Check sheet for the modelled part. Datum: model origin and axes. Units: mm. Face numbers are marked on the shaded views. A direction names the side the tool comes from. Round coordinates to 2 decimals unless told otherwise and drop trailing zeros. Write each loop counter-clockwise with the first axis right and the second up, starting at its lowest first coordinate (ties: lowest second). Pieces come first, ordered by that corner, then holes.
Item 1: Set-up check for the marked faces 1, 2, 3 and 4: record each of +Z, -Z, +X, -X, +Y, -Y from which the full face is reachable in a straight line by a thin tool's end or side.
Item 2: Section check B-B, the plane z = 10. State how many separate pieces and enclosed holes the cut face has, plus the area to 3 significant figures.
Item 3: Section check C-C, the plane y = -13. Record the cut outline in (x, z), plus the area to 3 significant figures.
Item 4: Material ranges on line 1 along Z through (x, y) = (24, 8.3); line 2 along Y through (x, z) = (-11, 18.75); line 3 along Y through (x, z) = (-6.5, 9.5), recorded low to high.
Item 5: Section check D-D, the plane x = 16. Record the cut outline in (y, z), plus the area to 3 significant figures.
Item 6: Release check for a two-part mould opening along Y. For the marked faces 5, 6 and 7 record: pulls with the +Y half, pulls with the -Y half, needs draft (parallel to the pull), parting line crosses it, or undercut.
Item 7: Section check A-A, the plane x = 24. Record the cut outline in (y, z), plus the area to 3 significant figures.
Item 8: Depth check by flat-ended pin: pin 1 (5.5 mm diameter, centred on x = 24, z = 9.5, fed in from -Y); pin 2 (10 mm diameter, centred on y = 11.5, z = 14, fed in from -X); pin 3 (2 mm diameter, centred on y = 18, z = 7.5, fed in from -X); pin 4 (5.5 mm diameter, centred on x = 24.5, z = 8.5, fed in from +Y). Enter the tip coordinate at first touch or a pass-through.
from build123d import *

# Parameters (mm, degrees)
SKETCH1_W           = 6.8
SKETCH1_H           = 2
SKETCH1_W_2         = 40
SKETCH1_H_2         = 39
BOSS_EXTRUDE1_DEPTH = 20
SKETCH2_R           = 4.5
BOSS_EXTRUDE2_DEPTH = 2
SKETCH3_R           = 5
BOSS_EXTRUDE3_DEPTH = 1.9
SKETCH4_R           = 3
BOSS_EXTRUDE4_DEPTH = 4
SKETCH5_R           = 10
BOSS_EXTRUDE5_DEPTH = 2
SKETCH6_R           = 2
CUT_EXTRUDE1_DEPTH  = 10
SKETCH7_R           = 2
CUT_EXTRUDE2_DEPTH  = 10
CUT_EXTRUDE3_DEPTH  = 5


with BuildPart() as part:
    # Sketch1 → Boss-Extrude1 (new body)
    with BuildSketch(Plane.XY):
        with Locations((-23.4, 7.722986842)):
            Rectangle(SKETCH1_W, SKETCH1_H)
        with Locations((0, -1.777013158)):
            Rectangle(SKETCH1_W_2, SKETCH1_H_2)
        with Locations((23.4, 7.722986842)):
            Rectangle(SKETCH1_W, SKETCH1_H)
    extrude(amount=BOSS_EXTRUDE1_DEPTH)

    # Sketch2 → Boss-Extrude2 (add)
    with BuildSketch(Plane(origin=(0, 17.722986842, 0), x_dir=(1, 0, 0), z_dir=(0, 1, 0))):
        with Locations(Location((-10, -10, 0), (0, 0, 180))):
            Circle(SKETCH2_R)
    extrude(amount=BOSS_EXTRUDE2_DEPTH)

    # Sketch3 → Boss-Extrude3 (add)
    with BuildSketch(Plane(origin=(0, 17.722986842, 0), x_dir=(1, 0, 0), z_dir=(0, 1, 0))):
        with Locations((-10, -10)):
            Circle(SKETCH3_R)
    extrude(amount=BOSS_EXTRUDE3_DEPTH)

    # Sketch4 → Boss-Extrude4 (add)
    with BuildSketch(Plane(origin=(0, 19.722986842, 0), x_dir=(1, 0, 0), z_dir=(0, 1, 0))):
        with Locations(Location((-10, -10, 0), (0, 0, 180))):
            Circle(SKETCH4_R)
    extrude(amount=BOSS_EXTRUDE4_DEPTH)

    # Sketch5 → Boss-Extrude5 (add)
    with BuildSketch(Plane(origin=(0, 23.722986842, 0), x_dir=(1, 0, 0), z_dir=(0, 1, 0))):
        with Locations(Location((-10, -10, 0), (0, 0, 180))):
            Circle(SKETCH5_R)
    extrude(amount=BOSS_EXTRUDE5_DEPTH)

    # Sketch6 → Cut-Extrude1 (cut)
    with BuildSketch(Plane(origin=(0, 8.722986842, 0), x_dir=(1, 0, 0), z_dir=(0, 1, 0))):
        with Locations(Location((24, -4, 0), (0, 0, 180))):
            Circle(SKETCH6_R)
        with Locations(Location((24, -16, 0), (0, 0, 180))):
            Circle(SKETCH6_R)
    extrude(amount=-CUT_EXTRUDE1_DEPTH, mode=Mode.SUBTRACT)

    # Sketch7 → Cut-Extrude2 (cut)
    with BuildSketch(Plane(origin=(0, 8.722986842, 0), x_dir=(1, 0, 0), z_dir=(0, 1, 0))):
        with Locations(Location((-24, -4, 0), (0, 0, 180))):
            Circle(SKETCH7_R)
        with Locations(Location((-24, -16, 0), (0, 0, 180))):
            Circle(SKETCH7_R)
    extrude(amount=-CUT_EXTRUDE2_DEPTH, mode=Mode.SUBTRACT)

    # Sketch8 → Cut-Extrude3 (cut)
    with BuildSketch(Plane(origin=(0, 25.722986842, 0), x_dir=(1, 0, 0), z_dir=(0, 1, 0))):
        with BuildLine():
            ThreePointArc((-18, -10), (-17, -11), (-16, -10))
            Line((-16, -10), (-18, -10))
        make_face()
        with BuildLine():
            Line((-18, -10), (-16, -10))
            ThreePointArc((-16, -10), (-17, -9), (-18, -10))
        make_face()
        with BuildLine():
            ThreePointArc((-10, -2), (-11, -3), (-10, -4))
            Line((-10, -4), (-10, -2))
        make_face()
        with BuildLine():
            Line((-10, -2), (-10, -4))
            ThreePointArc((-10, -4), (-9.292893219, -3.707106781), (-9, -3))
            ThreePointArc((-9, -3), (-9.292893219, -2.292893219), (-10, -2))
        make_face()
        with BuildLine():
            ThreePointArc((-2, -10), (-3, -9), (-4, -10))
            Line((-4, -10), (-2, -10))
        make_face()
        with BuildLine():
            Line((-2, -10), (-4, -10))
            ThreePointArc((-4, -10), (-3, -11), (-2, -10))
        make_face()
        with BuildLine():
            ThreePointArc((-9, -17), (-9.292893219, -16.292893219), (-10, -16))
            Line((-10, -16), (-10, -18))
            ThreePointArc((-10, -18), (-9.292893219, -17.707106781), (-9, -17))
        make_face()
        with BuildLine():
            Line((-10, -18), (-10, -16))
            ThreePointArc((-10, -16), (-11, -17), (-10, -18))
        make_face()
    extrude(amount=-CUT_EXTRUDE3_DEPTH, mode=Mode.SUBTRACT)


solid = part.part
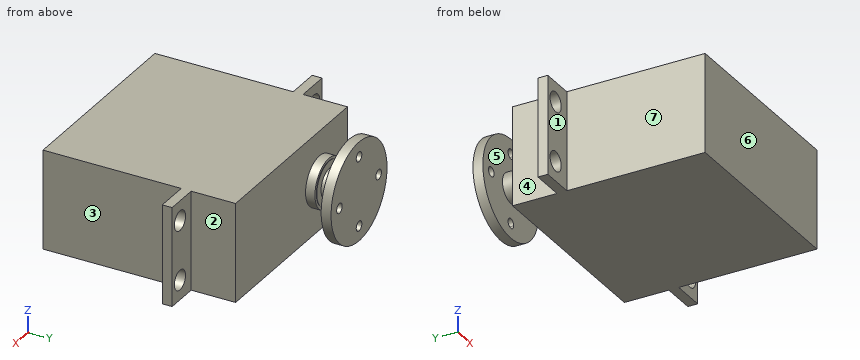
Values found:
1. face 1: +Z, -Z, -X, -Y
1. face 2: +Z, -Z, +X, +Y
1. face 3: +Z, -Z, +X, -Y
1. face 4: +Z, -Z, -X, +Y
2. separate pieces: 3
2. enclosed holes: 0
2. area: 1,660 mm2
3. outline: (-20, 0) - (20, 0) - (20, 20) - (-20, 20) - close
3. area: 800 mm2
4. line 1: z = 0 to 2, 6 to 14, 18 to 20
4. line 2: y = -21.28 to 17.72, 23.72 to 25.72
4. line 3: y = -21.28 to 19.72, 23.72 to 25.72
5. outline: (-21.28, 0) - (17.72, 0) - (17.72, 20) - (-21.28, 20) - close
5. area: 780 mm2
6. face 5: undercut
6. face 6: pulls with the -Y half
6. face 7: needs draft
7. outline: (6.72, 0) - (8.72, 0) - (8.72, 2) - (6.72, 2) - close; (6.72, 6) - (8.72, 6) - (8.72, 14) - (6.72, 14) - close; (6.72, 18) - (8.72, 18) - (8.72, 20) - (6.72, 20) - close
7. area: 24.0 mm2
8. pin 1: stops at y = 6.72
8. pin 2: stops at x = -26.8
8. pin 3: stops at x = -20
8. pin 4: stops at y = 8.72
